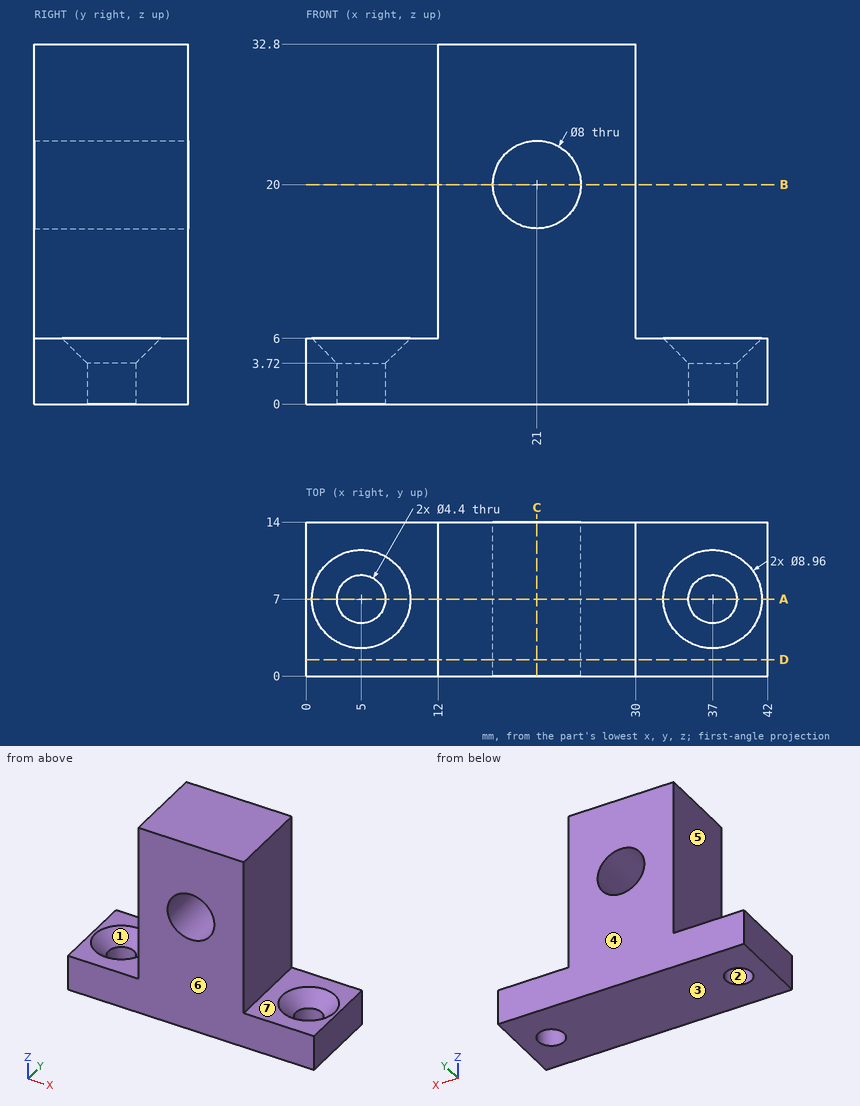
Design review of the part shown in the three views and the two pictorial views. Dimensions are in mm from the part's minimum x, y and z. A direction names the side the tool comes from. Coordinates: 2 decimals unless noted, no trailing zeros. Loops run counter-clockwise (first coordinate to the right, second up) from the corner with the lowest first, then second, coordinate; pieces in that order, holes last. Notation, with made-up numbers: M 51,39.5 L 103,39.5 A23 ccw 103,52.5 Z; hole C 86.5,68.25 d11. An arc over 180 degrees is marked long. Put each result on its own line as item: value. Start each with the question number.
Q1. Add section C-C (x = 21). Write out the cut boundary in (y, z), and give its area (3 significant figures).
Q2. Add section D-D (y = 1.5). Write out the cut boundary in (x, z).
Q3. Wall thickness on line 1 (X direction, y = 7, z = 2.8); line 2 (Y direction, x = 37, z = 2.95); line 3 (Z direction, x = 21, y = 10.5): over which ranges is each line inside the solid? List them lowest first.
Q4. Add section B-B (z = 20). Write out the cut boundary in (x, y), and give its area (3 significant figures).
Q5. Clearance check with flat-ended pins moving along their axes: pin 1 (4 mm diameter, centred on y = 7.5, z = 19, fed in from -X); pin 2 (10 mm diameter, centred on x = 24.5, z = 24, fed in from -Y); pin 3 (7 mm diameter, centred on y = 7.5, z = 22.5, fed in from +X). State where each tip first meets the part, or that it passes through.
Q6. The part is to be moulded in two halves that separate along Y. For the marked faces 1, 2, 3 and 4, say which applies: +Y half, -Y half, draft (parallel to the pull), parting line (faces both ways), or undercut.
Q7. For the marked faces 5, 6 and 7, list the 3-axis set-ups (+Z, -Z, +X, -X, +Y, -Y) from which the entire face can be reached by the end or side of a thin tool; tool diameter is ignored.
Q8. Add section A-A (y = 7). Write out the cut boundary in (x, z), and give its area (3 significant figures).
Answers:
1. outline: M 0,0 L 14,0 L 14,16 L 0,16 Z; M 0,24 L 14,24 L 14,32.8 L 0,32.8 Z
1. area: 347 mm^2
2. outline: M 0,0 L 42,0 L 42,6 L 30,6 L 30,32.8 L 12,32.8 L 12,6 L 0,6 Z; hole C 21,20 d8
3. line 1: x = 0 to 2.8, 7.2 to 34.8, 39.2 to 42
3. line 2: y = 0 to 4.8, 9.2 to 14
3. line 3: z = 0 to 16, 24 to 32.8
4. outline: M 12,0 L 17,0 L 17,14 L 12,14 Z; M 25,0 L 30,0 L 30,14 L 25,14 Z
4. area: 140 mm^2
5. pin 1: stops at x = 12
5. pin 2: stops at y = 0
5. pin 3: stops at x = 30
6. face 1: undercut
6. face 2: undercut
6. face 3: draft
6. face 4: +Y half
7. face 5: +Z, -X, +Y, -Y
7. face 6: +Z, -Z, +X, -X, -Y
7. face 7: +Z, +X, +Y, -Y
8. outline: M 0,0 L 2.8,0 L 2.8,3.72 L 0.52,6 L 0,6 Z; M 7.2,0 L 34.8,0 L 34.8,3.72 L 32.52,6 L 30,6 L 30,32.8 L 12,32.8 L 12,6 L 9.48,6 L 7.2,3.72 Z; M 39.2,0 L 42,0 L 42,6 L 41.48,6 L 39.2,3.72 Z; hole C 21,20 d8
8. area: 621 mm^2
